For this review, take the finished solid that the model builds, in its own axes (mm). Face numbers are marked on the shaded views. A direction names the side the tool comes from. Round coordinates to 2 decimals unless told otherwise and drop trailing zeros. Order: outer loops, then holes, each group sorted by start corner. A loop starts at its lowest first (then second) coordinate and runs counter-clockwise, first axis right, second up. Notation, with made-up numbers: (-30.75, -15.5) -> (-18.75, -15.5) arc R31 cw to (-18.75, 15.5) -> close; hole circle Ø2 at (-34, 6.5). An arc over 180 degrees is marked (long way). Use a Markdown table: item, result. Add a question column.
1) Clearance check with flat-ended pins moving along their axes: P1, Ø1.5, axis at x = 2, z = 7.5, coming from the -Y side; P2, Ø4, axis at x = 21.5, z = 5.5, coming from the -Y side; P3, Ø2, axis at x = -19.5, z = 5, coming from the -Y side. State where each tip first meets the part, or that it passes through.
2) Consider section A-A (x = -4.5). State the section outline as (y, z) points.
3) Machinability: for the marked faces 1, 2, 3, 4 and 5, which of the approach directions +Z, -Z, +X, -X, +Y, -Y give a long, thin tool a straight path to every point of the face, cutting with its end or side? Answer none if there is none.
4) Wall thickness on line 1 along Y through (x, z) = (-11.5, 8.5); line 2 along Y through (x, z) = (31, 1); line 3 along Y through (x, z) = (-30, 3.5): over which ranges is each line inside the solid? List them lowest first. Write a range as [from, to].
5) Consider section D-D (y = -3). State the section outline as (x, z) points, plus the area to 3 significant figures.
6) Consider section B-B (z = 6). State the section outline as (x, y) points.
7) Draft analysis for pull direction Y (two halves, no side actions). For the marked faces 6, 7, 8 and 9, state which applies: pulls with the +Y half, pulls with the -Y half, needs draft (parallel to the pull), parting line crosses it, or undercut.
8) Consider section C-C (x = 18.5). State the section outline as (y, z) points, plus the area to 3 significant figures.
```python
from build123d import *

# Parameters (mm, degrees)
F1_DEPTH = 12.7


with BuildPart() as f1:
    # F0 (on Top) → F1 (new body)
    with BuildSketch(Plane.XY):
        Polygon((48.759662, 54.159728), (-42.306267, 54.159728), (-33.266246, 41.459728), (-2.446738, 41.459728), (-2.446738, 33.161538), (-21.345066, 33.161538), (-15.30465, 24.368381), (-2.446738, 24.368381), (-2.446738, 0), (-2.446738, -9.455727), (15.856527, 15.478381), (22.471367, 15.478381), (32.149471, 15.478381), (38.04643, 24.368381), (12.793262, 24.368381), (12.793262, 41.459728), (39.707991, 41.459728), align=None)
    extrude(amount=F1_DEPTH)


solid = f1.part
```
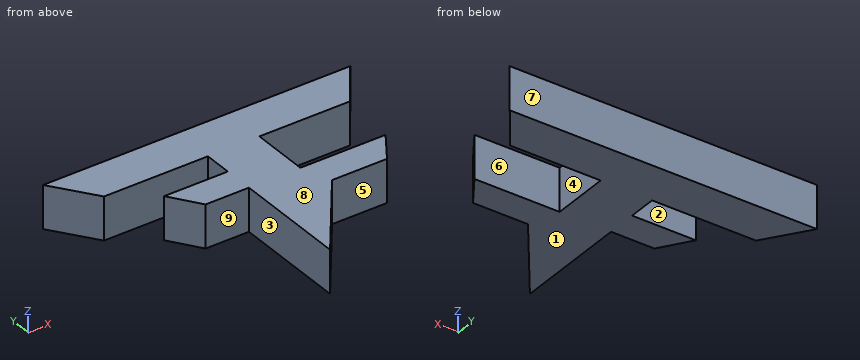
Results list:
| question | item | result |
|---|---|---|
| 1 | P1 | y = -4.42 |
| 1 | P2 | y = 15.48 |
| 1 | P3 | y = 29.02 |
| 2 | outline | (24.37, 0) -> (33.16, 0) -> (33.16, 12.7) -> (24.37, 12.7) -> close; (41.46, 0) -> (54.16, 0) -> (54.16, 12.7) -> (41.46, 12.7) -> close |
| 3 | face 1 | -Z, +X, -X, +Y, -Y |
| 3 | face 2 | +Z, -Z, -X |
| 3 | face 3 | +Z, -Z, -X, -Y |
| 3 | face 4 | +Z, -Z, +X |
| 3 | face 5 | +Z, -Z, +X, -Y |
| 4 | line 1 | [24.37, 33.16], [41.46, 54.16] |
| 4 | line 2 | [15.48, 24.37], [41.46, 54.16] |
| 4 | line 3 | [41.46, 54.16] |
| 5 | outline | (-2.45, 0) -> (2.29, 0) -> (2.29, 12.7) -> (-2.45, 12.7) -> close |
| 5 | area | 60.2 mm2 |
| 6 | outline | (-42.31, 54.16) -> (-33.27, 41.46) -> (-2.45, 41.46) -> (-2.45, 33.16) -> (-21.35, 33.16) -> (-15.3, 24.37) -> (-2.45, 24.37) -> (-2.45, -9.46) -> (15.86, 15.48) -> (32.15, 15.48) -> (38.05, 24.37) -> (12.79, 24.37) -> (12.79, 41.46) -> (39.71, 41.46) -> (48.76, 54.16) -> close |
| 7 | face 6 | undercut |
| 7 | face 7 | pulls with the +Y half |
| 7 | face 8 | needs draft |
| 7 | face 9 | pulls with the -Y half |
| 8 | outline | (15.48, 0) -> (24.37, 0) -> (24.37, 12.7) -> (15.48, 12.7) -> close; (41.46, 0) -> (54.16, 0) -> (54.16, 12.7) -> (41.46, 12.7) -> close |
| 8 | area | 274 mm2 |
